```python
from build123d import *

# Parameters (mm, degrees)
BOSS_EXTRUDE1_DEPTH = 3
SKETCH3_W           = 10
SKETCH3_H           = 3
BOSS_EXTRUDE2_DEPTH = 25
SKETCH4_W           = 3
SKETCH4_H           = 22.5
BOSS_EXTRUDE3_DEPTH = 25


with BuildPart() as part:
    # Sketch2 → Boss-Extrude1 (new body)
    with BuildSketch(Plane(origin=(0, 0, 0), x_dir=(1, 0, 0), z_dir=(0, 1, 0))):
        with BuildLine():
            Line((26.055569119, 8.188046441), (26.055569119, -22.896953559))
            Line((26.055569119, -22.896953559), (-26.055569119, -22.896953559))
            Line((-26.055569119, -22.896953559), (-26.055569119, 8.188046441))
            ThreePointArc((-26.055569119, 8.188046441), (-21.514872246, 4.669726518), (-15.870079226, 5.73406431))
            ThreePointArc((-15.870079226, 5.73406431), (-10.616247764, 4.133629141), (-7, 0))
            ThreePointArc((-7, 0), (0, -7), (7, 0))
            ThreePointArc((7, 0), (10.616247764, 4.133629141), (15.870079226, 5.73406431))
            ThreePointArc((15.870079226, 5.73406431), (21.514872246, 4.669726518), (26.055569119, 8.188046441))
        make_face()
    extrude(amount=BOSS_EXTRUDE1_DEPTH)

    # Sketch3 → Boss-Extrude2 (add)
    with BuildSketch(Plane.XY.offset(22.896953559)):
        with Locations((-21.055569119, 1.5)):
            Rectangle(SKETCH3_W, SKETCH3_H)
    extrude(amount=BOSS_EXTRUDE2_DEPTH)

    # Sketch4 → Boss-Extrude3 (add)
    with BuildSketch(Plane.XZ):
        with Locations((-24.555569119, 36.646953559)):
            Rectangle(SKETCH4_W, SKETCH4_H)
    extrude(amount=BOSS_EXTRUDE3_DEPTH)


solid = part.part
```
The model under review builds one solid part; all positions refer to its coordinate system, in mm. A direction names the side the tool comes from. Round coordinates to 2 decimals unless told otherwise and drop trailing zeros. Loops run counter-clockwise (first coordinate to the right, second up) from the corner with the lowest first, then second, coordinate; pieces in that order, holes last. Notation, with made-up numbers: (0.25, 53) -> (52.25, 53) arc R32 ccw to (52.25, 83) -> close; hole circle Ø7 at (70, 60.5). An arc over 180 degrees is marked (long way). Answer in a Markdown table with one row per item.
1) Consider section B-B, the plane z = 39.5. Write out the cut boundary in (x, y), plus the area to 3 significant figures.
Taken from the geometry:
| item | result |
|---|---|
| outline | (-26.06, -25) -> (-23.06, -25) -> (-23.06, 0) -> (-16.06, 0) -> (-16.06, 3) -> (-26.06, 3) -> close |
| area | 105 mm² |
2) Draft analysis for pull direction X (two halves, no side actions). For faces 1 (the flat face through (-23.3, -7.7, 47.897)), 2 (the flat face through (-16.056, 1, 35)), 3 (the flat face through (-26.056, -11, 32)), 4 (the cylindrical face through (21.43, 1.48, -4.65)), state which applies: pulls with the +X half, pulls with the -X half, needs draft (parallel to the pull), parting line crosses it, or undercut.
Taken from the geometry:
| item | result |
|---|---|
| face 1 | needs draft |
| face 2 | pulls with the +X half |
| face 3 | pulls with the -X half |
| face 4 | undercut |
3) Consider section C-C, the plane y = -22.75. Write out the cut boundary in (x, z).
Taken from the geometry:
| item | result |
|---|---|
| outline | (-26.06, 25.4) -> (-23.06, 25.4) -> (-23.06, 47.9) -> (-26.06, 47.9) -> close |
4) Tool access review of faces 5 (the flat face through (-23.056, -12, 36)), 6 (the flat face through (5, 1, 22.897)), 7 (the cylindrical face through (10.55, 1.48, -4.09)), 8 (the flat face through (-25, -12, 25.397)): name each direction out of +Z, -Z, +X, -X, +Y, -Y from which nothing blocks a thin tool from reaching the whole face with its end or side.
Taken from the geometry:
| item | result |
|---|---|
| face 5 | +Z, -Z, +X, -Y |
| face 6 | +Z, +X, +Y, -Y |
| face 7 | -Z, +Y, -Y |
| face 8 | -Z, +X, -X, -Y |
5) For pin 1 Ø8 at (y, z) = (0, 36) entering from +X; pin 2 Ø15.5 at (x, z) = (10.5, 30.5) entering from -Y; pin 3 Ø0.9 at (x, y) = (-24, -8.5) entering from -Z, all flat-tipped, find the tip position at first contact; note any pin that passes through.
Taken from the geometry:
| item | result |
|---|---|
| pin 1 | stops at x = -16.06 |
| pin 2 | stops at y = 0 |
| pin 3 | stops at z = 25.4 |
6) Wall thickness on line 1 along Y through (x, z) = (2.5, 8.5); line 2 along X through (y, z) = (-9.75, 28); line 3 along Z through (x, y) = (6, 1.75): over which ranges is each line inside the solid? List them lowest first.
Taken from the geometry:
| item | result |
|---|---|
| line 1 | y = 0 to 3 |
| line 2 | x = -26.06 to -23.06 |
| line 3 | z = 3.61 to 22.9 |
7) Consider section A-A, the plane z = -3.5. Write out the cut boundary in (x, y).
Taken from the geometry:
| item | result |
|---|---|
| outline | (-26.06, 0) -> (-9.74, 0) -> (-9.74, 3) -> (-26.06, 3) -> close; (9.74, 0) -> (26.06, 0) -> (26.06, 3) -> (9.74, 3) -> close |
8) Consider section D-D, the plane x = 0. Write out the cut boundary in (y, z).
Taken from the geometry:
| item | result |
|---|---|
| outline | (0, 7) -> (3, 7) -> (3, 22.9) -> (0, 22.9) -> close |
